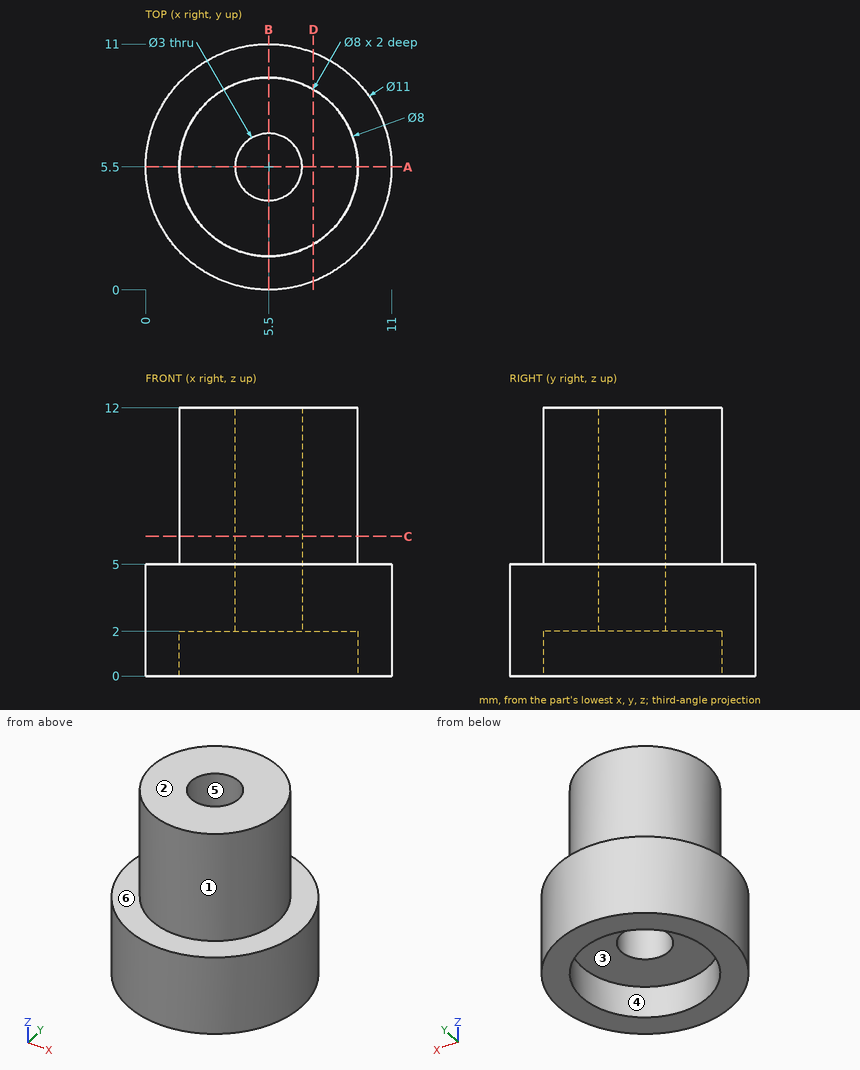
Can you work these out from the drawing? Everything is in mm from the part's minimum corner. A direction names the side the tool comes from. Coordinates: 2 decimals unless noted, no trailing zeros. Write each loop counter-clockwise with the first axis right and the second up, starting at its lowest first coordinate (ties: lowest second). Pieces come first, ordered by that corner, then holes. Notation, with made-up numbers: (-13.5, 51) -> (25.5, 51) arc R29 ccw to (25.5, 87) -> close; hole circle Ø9 at (75, 15.5). An arc over 180 degrees is marked (long way). Write item = value, one per line.
(1) Imagine slicing it at C-C (z = 6.25). Please give me the cut outline in (x, y), and give its area (3 significant figures).
Verdict:
outline = circle Ø8 at (5.5, 5.5); hole circle Ø3 at (5.5, 5.5)
area = 43.2 mm^2
(2) On a 3-axis mill with a long thin cutter (end or side, diameter ignored), from which of +Z, -Z, +X, -X, +Y, -Y can I reach the whole of each face in a straight line? I mean the marked faces 4, 5 and 6. Say none if no direction works.
Verdict:
face_4 = -Z
face_5 = +Z, -Z
face_6 = +Z
(3) Imagine slicing it at D-D (x = 7.5). Please give me the cut outline in (y, z), and give its area (3 significant figures).
Verdict:
outline = (0.38, 0) -> (2.04, 0) -> (2.04, 2) -> (8.96, 2) -> (8.96, 0) -> (10.62, 0) -> (10.62, 5) -> (8.96, 5) -> (8.96, 12) -> (2.04, 12) -> (2.04, 5) -> (0.38, 5) -> close
area = 85.9 mm^2
(4) Imagine slicing it at A-A (y = 5.5). Please give me the cut outline in (x, z).
Verdict:
outline = (0, 0) -> (1.5, 0) -> (1.5, 2) -> (4, 2) -> (4, 12) -> (1.5, 12) -> (1.5, 5) -> (0, 5) -> close; (7, 2) -> (9.5, 2) -> (9.5, 0) -> (11, 0) -> (11, 5) -> (9.5, 5) -> (9.5, 12) -> (7, 12) -> close
(5) If I drill on probe 1 along Y at (x, z) = (5.5, 0.85); probe 2 along Y at (x, z) = (5.5, 6.75); probe 3 along Z at (x, y) = (10.25, 8), over which ranges is the centre line in solid material (lowest first)?
Verdict:
probe_1 = 0 to 1.5, 9.5 to 11
probe_2 = 1.5 to 4, 7 to 9.5
probe_3 = 0 to 5
(6) For pin 1 (1 mm diameter, centred on y = 3.5, z = 9.5, fed in from +X); pin 2 (5 mm diameter, centred on x = 5.5, y = 5.5, fed in from +Z); pin 3 (5 mm diameter, centred on x = 5.5, y = 5.5, fed in from -Z); pin 4 (5 mm diameter, centred on y = 3.5, z = 9.5, fed in from -X), each with a flat end and sliding along its axis, tell me the tip position at first contact or that it passes through.
Verdict:
pin_1 = 9.21
pin_2 = 12
pin_3 = 2
pin_4 = 1.5
(7) Thinking about a two-plate mould opening in X: for the marked faces 1, 2 and 3, which applies, +X half, -X half, draft (parallel to the pull), parting line (faces both ways), or undercut?
Verdict:
face_1 = parting line
face_2 = draft
face_3 = undercut
